Could you check a few things on this model? Use its own coordinates, in mm. A direction names the side the tool comes from. Round coordinates to 2 decimals unless told otherwise and drop trailing zeros. Write each loop counter-clockwise with the first axis right and the second up, starting at its lowest first coordinate (ties: lowest second). Pieces come first, ordered by that corner, then holes. Notation, with made-up numbers: (-23.75, 76.25) - (9.25, 76.25) arc R18 ccw to (9.25, 95.25) - close; hole circle Ø7 at (26, -34.75). An arc over 180 degrees is marked (long way). Put each result on its own line as item: value.
from build123d import *

# Parameters (mm, degrees)
SKETCH1_W           = 80
SKETCH1_H           = 50
BOSS_EXTRUDE1_DEPTH = 2.4
SKETCH2_W           = 74.5
SKETCH2_H           = 44.5
BOSS_EXTRUDE2_DEPTH = 1.8
SKETCH4_R           = 9.6
SKETCH4_R_2         = 14
SKETCH4_R_3         = 2.25
CUT_EXTRUDE1_DEPTH  = 95.013072971
BOSS_EXTRUDE3_DEPTH = 74.5
FILLET1_R           = 3
FILLET2_R           = 3
SKETCH7_R           = 3
CUT_EXTRUDE3_DEPTH  = 2.25
CHAMFER1_SIZE       = 3


with BuildPart() as part:
    # Sketch1 → Boss-Extrude1 (new body)
    with BuildSketch(Plane(origin=(0, 0, 0), x_dir=(1, 0, 0), z_dir=(0, 1, 0))):
        with Locations((38.753665689, 26.173020528)):
            Rectangle(SKETCH1_W, SKETCH1_H)
    extrude(amount=BOSS_EXTRUDE1_DEPTH)

    # Sketch2 → Boss-Extrude2 (add)
    with BuildSketch(Plane(origin=(0, 2.4, 0), x_dir=(1, 0, 0), z_dir=(0, 1, 0))):
        with Locations((38.753665689, 26.173020528)):
            Rectangle(SKETCH2_W, SKETCH2_H)
    extrude(amount=BOSS_EXTRUDE2_DEPTH)

    # Sketch4 → Cut-Extrude1 (cut, through all)
    with BuildSketch(Plane(origin=(0, 0, 0), x_dir=(-1, 0, 0), z_dir=(0, -1, 0))):
        with Locations(Location((-65.718665689, 28.723020528, 0), (0, 0, 90))):
            Circle(SKETCH4_R)
        with Locations(Location((-38.753665689, 28.723020528, 0), (0, 0, 90))):
            Circle(SKETCH4_R_2)
        with Locations(Location((-11.788665689, 28.723020528, 0), (0, 0, 90))):
            Circle(SKETCH4_R)
        with Locations(Location((-72.753665689, 7.173020528, 0), (0, 0, 90))):
            Circle(SKETCH4_R_3)
        with Locations(Location((-4.753665689, 7.173020528, 0), (0, 0, 90))):
            Circle(SKETCH4_R_3)
    extrude(amount=-CUT_EXTRUDE1_DEPTH, mode=Mode.SUBTRACT)

    # Sketch5 → Boss-Extrude3 (add)
    with BuildSketch(Plane(origin=(76.003665689, 0, 0), x_dir=(0, 0, -1), z_dir=(1, 0, 0))):
        Polygon((48.123020528, 4.2), (44.123020528, 4.2), (44.373020528, 8.2), (50.373020528, 8.2), (50.373020528, 7.1), (48.142477117, 4.978263585), align=None)
    extrude(amount=-BOSS_EXTRUDE3_DEPTH)

    # Fillet1
    fillet1_edges = [part.edges().sort_by_distance(p)[0] for p in [
        (-1.246334311, 1.2, -51.173020528),
        (78.753665689, 1.2, -51.173020528),
        (78.753665689, 1.2, -1.173020528),
        (-1.246334311, 1.2, -1.173020528),
    ]]
    fillet(fillet1_edges, radius=FILLET1_R)

    # Fillet2
    # the kernel refuses this fillet: 3 mm, written as the material it takes off along each edge
    with BuildSketch(Plane(origin=(1.753665689, 0, -48.173020528), x_dir=(-1, 0, 0), z_dir=(0, 0, 1))) as fillet2_piece_1:
        with BuildLine():
            CenterArc((0.060612309, -3), FILLET2_R, 11.536959033, 78.463040967)
            Line((3, -2.4), (3.058787754, -2.388))
            ThreePointArc((3.058787754, -2.388), (3.06, -1.2), (3.06, 0))
            Line((3.06, 0), (3, 0.06))
            Line((3, 0.06), (0.060612309, 0.06))
            Line((0.060612309, 0.06), (0.060612309, 0))
        make_face()
    revolve(axis=Axis((1.753665689, 0, -48.173020528), (0, -1, 0)), revolution_arc=90, mode=Mode.SUBTRACT)
    with BuildSketch(Plane(origin=(75.753665689, 0, -51.173020528), x_dir=(0, 0, 1), z_dir=(-1, 0, 0))) as fillet2_piece_2:
        with BuildLine():
            CenterArc((2.939387691, 3), FILLET2_R, 191.536959033, 78.463040967)
            Line((0, 2.4), (-0.058787754, 2.388))
            ThreePointArc((-0.058787754, 2.388), (-0.06, 1.2), (-0.06, 0))
            Line((-0.06, 0), (0, -0.06))
            Line((0, -0.06), (2.939387691, -0.06))
            Line((2.939387691, -0.06), (2.939387691, 0))
        make_face()
    extrude(amount=74, mode=Mode.SUBTRACT)
    with BuildSketch(Plane(origin=(75.753665689, 0, -48.173020528), x_dir=(1, 0, 0), z_dir=(0, 0, 1))) as fillet2_piece_3:
        with BuildLine():
            CenterArc((0.060612309, 3), FILLET2_R, 270, 78.463040967)
            Line((3, 2.4), (3.058787754, 2.388))
            ThreePointArc((3.058787754, 2.388), (3.06, 1.2), (3.06, 0))
            Line((3.06, 0), (3, -0.06))
            Line((3, -0.06), (0.060612309, -0.06))
            Line((0.060612309, -0.06), (0.060612309, 0))
        make_face()
    revolve(axis=Axis((75.753665689, 0, -48.173020528), (0, 1, 0)), revolution_arc=90, mode=Mode.SUBTRACT)
    with BuildSketch(Plane(origin=(78.753665689, 0, -4.173020528), x_dir=(-1, 0, 0), z_dir=(0, 0, -1)), Plane(origin=(-1.246334311, 0, -48.173020528), x_dir=(1, 0, 0), z_dir=(0, 0, 1))) as fillet2_piece_4:
        with BuildLine():
            CenterArc((2.939387691, 3), FILLET2_R, 191.536959033, 78.463040967)
            Line((0, 2.4), (-0.058787754, 2.388))
            ThreePointArc((-0.058787754, 2.388), (-0.06, 1.2), (-0.06, 0))
            Line((-0.06, 0), (0, -0.06))
            Line((0, -0.06), (2.939387691, -0.06))
            Line((2.939387691, -0.06), (2.939387691, 0))
        make_face()
    extrude(amount=44, mode=Mode.SUBTRACT)
    with BuildSketch(Plane(origin=(75.753665689, 0, -4.173020528), x_dir=(0, 0, 1), z_dir=(-1, 0, 0))) as fillet2_piece_5:
        with BuildLine():
            CenterArc((0.060612309, 3), FILLET2_R, 270, 78.463040967)
            Line((3, 2.4), (3.058787754, 2.388))
            ThreePointArc((3.058787754, 2.388), (3.06, 1.2), (3.06, 0))
            Line((3.06, 0), (3, -0.06))
            Line((3, -0.06), (0.060612309, -0.06))
            Line((0.060612309, -0.06), (0.060612309, 0))
        make_face()
    revolve(axis=Axis((75.753665689, 0, -4.173020528), (0, 1, 0)), revolution_arc=90, mode=Mode.SUBTRACT)
    with BuildSketch(Plane(origin=(1.753665689, 0, -1.173020528), x_dir=(0, 1.0, -1.5658770576478976e-12), z_dir=(1, 0, 0))) as fillet2_piece_6:
        with BuildLine():
            CenterArc((3, -2.939387691), FILLET2_R, 101.536959033, 78.463040967)
            Line((0, -2.939387691), (-0.06, -2.939387691))
            Line((-0.06, -2.939387691), (-0.06, 0))
            Line((-0.06, 0), (0, 0.06))
            ThreePointArc((0, 0.06), (1.2, 0.06), (2.388, 0.058787754))
            Line((2.388, 0.058787754), (2.4, 0))
        make_face()
    extrude(amount=74, mode=Mode.SUBTRACT)
    with BuildSketch(Plane(origin=(1.753665689, 0, -4.173020528), x_dir=(0, 0, 1), z_dir=(1, 0, 0))) as fillet2_piece_7:
        with BuildLine():
            CenterArc((0.060612309, -3), FILLET2_R, 11.536959033, 78.463040967)
            Line((3, -2.4), (3.058787754, -2.388))
            ThreePointArc((3.058787754, -2.388), (3.06, -1.2), (3.06, 0))
            Line((3.06, 0), (3, 0.06))
            Line((3, 0.06), (0.060612309, 0.06))
            Line((0.060612309, 0.06), (0.060612309, 0))
        make_face()
    revolve(axis=Axis((1.753665689, 0, -4.173020528), (0, -1, 0)), revolution_arc=90, mode=Mode.SUBTRACT)

    # Sketch7 → Cut-Extrude3 (cut)
    with BuildSketch(Plane.XZ):
        with Locations(Location((4.753665689, -7.173020528, 0), (0, 0, 270))):
            Circle(SKETCH7_R)
        with Locations(Location((72.753665689, -7.173020528, 0), (0, 0, 270))):
            Circle(SKETCH7_R)
    extrude(amount=-CUT_EXTRUDE3_DEPTH, mode=Mode.SUBTRACT)

    # Chamfer1
    # the kernel refuses this chamfer: 3 mm, written as the material it takes off along each edge
    with BuildSketch(Plane(origin=(11.788665689, 4.2, -28.723020528), x_dir=(0, 0, -1), z_dir=(-1, 0, 0))) as chamfer1_piece_1:
        Polygon((9.6 + CHAMFER1_SIZE, 0), (9.6, CHAMFER1_SIZE), (9.6, 0), align=None)
    revolve(axis=Axis((11.788665689, 4.2, -28.723020528), (0, -1, 0)), mode=Mode.SUBTRACT)
    with BuildSketch(Plane(origin=(38.753665689, 4.2, -28.723020528), x_dir=(0, 0, -1), z_dir=(-1, 0, 0))) as chamfer1_piece_2_section:
        Polygon((14 + CHAMFER1_SIZE, 0), (14, CHAMFER1_SIZE), (14, 0), align=None)
    chamfer1_piece_2 = revolve(axis=Axis((38.753665689, 4.2, -28.723020528), (0, -1, 0)), mode=Mode.PRIVATE)
    chamfer1_piece_2 = split(chamfer1_piece_2, bisect_by=Plane(origin=(38.753665689, 0.839630842, -43.912997455), z_dir=(0, 0.06237828615517877, 0.9980525784828888)), keep=Keep.TOP, mode=Mode.PRIVATE)
    add(chamfer1_piece_2, mode=Mode.SUBTRACT)
    with BuildSketch(Plane(origin=(65.718665689, 4.2, -28.723020528), x_dir=(0, 0, -1), z_dir=(-1, 0, 0))) as chamfer1_piece_3:
        Polygon((9.6 + CHAMFER1_SIZE, 0), (9.6, CHAMFER1_SIZE), (9.6, 0), align=None)
    revolve(axis=Axis((65.718665689, 4.2, -28.723020528), (0, -1, 0)), mode=Mode.SUBTRACT)


solid = part.part
(1) Please list where these lines run through material, in increasing order: probe 1 along X at (y, z) = (3, -7); probe 2 along X at (y, z) = (0.75, -36); probe 3 along X at (y, z) = (2, -41.5). Write a range as from..to.
Values found:
probe 1: x = 1.5..2.51, 7..70.51, 75..76
probe 2: x = -0.29..5.53, 18.05..26.79, 50.71..59.46, 71.98..77.8
probe 3: x = -1.14..31.28, 46.22..78.64
(2) I'm going to push flat-ended pins straight in: pin 1 (3 mm diameter, centred on x = 25.5, z = -18.5, fed in from +Y); pin 2 (2 mm diameter, centred on x = 28.5, y = 3.5, fed in from -Z); pin 3 (5.5 mm diameter, centred on x = 4.75, z = -7.17, fed in from -Y). Where does each tip first touch, or does it pass through?
Values found:
pin 1: stops at y = 4.2
pin 2: stops at z = -48.42
pin 3: stops at y = 2.25
(3) Imagine slicing it at A-A, the plane z = -7. List the corners of the cut face in (x, y) for me, then the cut area to 3 significant figures.
Values found:
outline: (-1.25, 2.4) arc R3 ccw to (1.69, 0) - (1.76, 0) - (1.76, 2.25) - (2.51, 2.25) - (2.51, 4.2) - (1.5, 4.2) - (1.5, 2.4) - close; (7, 2.25) - (7.75, 2.25) - (7.75, 0) - (69.76, 0) - (69.76, 2.25) - (70.51, 2.25) - (70.51, 4.2) - (7, 4.2) - close; (75, 2.25) - (75.75, 2.25) - (75.75, 0) - (75.81, 0) arc R3 ccw to (78.75, 2.4) - (76, 2.4) - (76, 4.2) - (75, 4.2) - close
area: 278 mm^2
(4) Imagine slicing it at B-B, the plane z = -26.5. Give the number of separate pieces and of enclosed holes in the cut face, then the cut area to 3 significant figures.
Values found:
separate pieces: 4
enclosed holes: 0
area: 28.9 mm^2
(5) If we mould it in two halves opening along Y, with no side actions, what happens to faces 5 (the face through (2.417, 0.592, -26.642)), 6 (the face through (39.28, 5.94, -44.23)), 7 (the face through (39, 2.4, -49)), 8 (the face through (38, 3, -48.423))? For each: pulls with the +Y half, pulls with the -Y half, needs draft (parallel to the pull), parting line crosses it, or undercut.
Values found:
face 5: needs draft
face 6: pulls with the +Y half
face 7: undercut
face 8: undercut
(6) For faces 1 (the face through (74.985, 3.211, -6.88)), 2 (the face through (16, 4.2, -42)), 3 (the face through (1.504, 4, -43)), 4 (the face through (7, 2.25, -6)), which set-ups out of +Z, -Z, +X, -X, +Y, -Y let a thin tool reach every point of the face, with its end or its side?
Values found:
face 1: +Y, -Y
face 2: +Z, +X, -X, +Y
face 3: +Z, -Z, -X, +Y
face 4: -Y
